Check sheet for the modelled part. Datum: model origin and axes. Units: mm. Round coordinates to 2 decimals unless told otherwise and drop trailing zeros. Write each loop counter-clockwise with the first axis right and the second up, starting at its lowest first coordinate (ties: lowest second). Pieces come first, ordered by that corner, then holes.
Autodesk Inventor part; units mm, degrees
ref_plane "YZ Plane" through (0, 0, 0) normal (1, 0, 0) x (0, 1, 0)
ref_plane "XZ Plane" through (0, 0, 0) normal (0, 1, 0) x (-1, 0, 0)
ref_plane "XY Plane" through (0, 0, 0) normal (0, 0, 1) x (1, 0, 0)
sketch "Sketch1" plane through (0, 0, 0) normal (0, 0, 1) x (1, 0, 0)
  arc A0 (-19.4827, -3.287) -> (-19.05, 0) centre (-31.75, 0) ccw
  line L0 (-19.4827, -3.287) -> (-58.7375, -149.7878)
  line L1 (-65.8876, 46.8376) -> (-65.8876, 21.4376)
  line L2 (-65.8876, 21.4376) -> (-71.4375, 21.4376)
  line L3 (-44.45, 34.1376) -> (-38.6524, 34.1376)
  line L4 (-44.45, 34.1376) -> (0, 34.1376) construction
  line L5 (-37.3992, -46.4536) -> (-31.0492, -46.4536)
  line L6 (-71.4375, 21.4376) -> (-71.4375, 8.7376)
  line L7 (-71.4375, 8.7376) -> (-58.7375, 8.7376)
  line L8 (-58.7375, 8.7376) -> (-52.3875, 8.7376)
  line L9 (-52.3875, 8.7376) -> (-52.3875, -102.3907)
  line L10 (-71.4375, 8.7376) -> (-71.4375, -0.7874)
  line L11 (-71.4375, 8.7376) -> (-61.9125, 8.7376) construction
  line L12 (-71.4375, -0.7874) -> (-58.7375, -0.7874)
  line L13 (-58.7375, -0.7874) -> (-58.7375, -51.5874)
  line L14 (-58.7375, -51.5874) -> (-71.4375, -51.5874)
  line L15 (-71.4375, -0.7874) -> (-65.0875, -0.7874)
  line L16 (-65.0875, -0.7874) -> (-65.0875, -6.731)
  line L17 (-65.0875, -6.731) -> (-71.4375, -6.731)
  line L18 (-71.4375, 21.4376) -> (-71.4375, -0.7874)
  line L19 (-71.4375, -6.731) -> (-71.4375, -51.5874)
  line L20 (-58.7375, -51.5874) -> (-58.7375, -126.0892)
  line L21 (-58.7375, -51.5874) -> (0, -51.5874) construction
  line L22 (-46.0375, -102.3907) -> (-52.3875, -102.3907)
  line L23 (-65.0875, -51.5907) -> (-58.7375, -51.5907)
  line L24 (-58.7375, -149.7878) -> (-61.9125, -161.637)
  line L25 (-58.7375, -149.7878) -> (-34.203, -149.7878) construction
  line L26 (-65.0875, -161.637) -> (-61.9125, -161.637)
  line L27 (-58.7375, -126.0892) -> (-52.3875, -126.0892)
  line L28 (0, 34.1376) -> (0, 0)
  line L29 (-65.0875, -100.6892) -> (-65.0875, -161.637)
  line L30 (-58.7375, -51.5907) -> (-61.9125, -51.5907)
  line L31 (-65.0875, -100.6892) -> (-58.7375, -100.6892)
  line L32 (-65.8876, 46.8376) -> (-18.3062, 46.8376) construction
  line L33 (-65.8876, 46.8376) -> (-14.7047, 46.8376) construction
  line L34 (-65.8876, 46.8376) -> (-33.5957, 31.7796)
  line L35 (-65.8876, 46.8376) -> (-30.2574, 46.8376) construction
  arc A1 (-19.05, 0) -> (-33.5957, 31.7796) centre (-61.0391, 0) ccw
  line L36 (-44.45, 34.1376) -> (-44.45, -46.4536)
  line L37 (-44.45, 34.1376) -> (36.1412, 34.1376) construction
  line L38 (-44.45, -46.4536) -> (-37.3992, -46.4536)
  dimension "d56" = 19.05
  dimension "d57" = 25.4
  dimension "d58" = 5.5499
  dimension "d59" = 65.8876
  dimension "d60" = 12.7
  dimension "d61" = 12.7
  dimension "d62" = 44.45
  dimension "d63" = 6.35
  dimension "d64" = 105
  dimension "d65" = 12.7
  dimension "d66" = 12.7
  dimension "d67" = 6.35
  dimension "d68" = 9.525
  dimension "d69" = 50.8
  dimension "d70" = 12.7
  dimension "d71" = 6.35
  dimension "d72" = 5.9436
  dimension "d73" = 6.35
  dimension "d74" = 50.8
  dimension "d75" = 6.35
  dimension "d76" = 105
  dimension "d77" = 3.175
  dimension "d78" = 6.35
  dimension "d79" = 60.9478
  dimension "d80" = 3.175
  dimension "d81" = 6.35
  dimension "d82" = 25.4
  dimension "d83" = 25
  dimension "d84" = 41.9891
  dimension "d85" = 32.2919
  dimension "d86" = 90
  dimension "d87" = 80.5912
revolve "Revolution1" add sketch "Sketch1" angle 360 about axis through (0, 34.1376, 0) along (0, -1, 0) contours L0 L5 L38 L36 L3 L34 A1 A0
properties part number "Graphite" material "GFRC"
1. Sectioned sample at D-D, the plane y = 20. Enter the section's corners in (x, z), plus the area to 3 significant figures.
2. Sectioned sample at B-B, the plane x = 0. Enter the section's corners in (y, z), plus the area to 3 significant figures.
3. Sectioned sample at C-C, the plane y = -7. Enter the section's corners in (x, z).
4. Release check for a two-part mould opening along Z. For faces 1 (the conical face through (5.2, -20.4, 23.5)), 2 (the cylindrical face through (-42.397, -6.722, -13.352)), 3 (the flat face through (30, -46.454, 9)) record: released by +Z, released by -Z, zero draft, split by the parting line, or undercut.
5. Go/stop test with flat-tipped pins: pin 1 (4 mm diameter, centred on y = -10, z = -15, fed in from -X); pin 2 (1 mm diameter, centred on x = 28.5, y = -36, fed in from -Z); pin 3 (4 mm diameter, centred on x = -21.5, y = -13, fed in from -Z); pin 4 (1.5 mm diameter, centred on x = -35, z = 15, fed in from +Y). Record where each tip stops, or that it passes through.
6. Sectioned sample at A-A, the plane z = 0. Enter the section's corners in (x, y), plus the area to 3 significant figures.
7. Scan lines: line 1 along Z through (x, y) = (-3.5, 1.5); line 2 along Z through (x, y) = (-5.5, -9); line 3 along X through (y, z) = (-23, 11). Record each from-to range of solid material in increasing order.
Computed values:
1. outline: circle Ø88.9 at (0, 0); hole circle Ø48.24 at (0, 0)
1. area: 4,380 mm2
2. outline: (-46.45, -44.45) - (34.14, -44.45) - (34.14, -38.65) - (31.78, -33.6) arc R41.99 ccw to (0, -19.05) arc R12.7 ccw to (-3.29, -19.48) - (-46.45, -31.05) - close; (-46.45, 31.05) - (-3.29, 19.48) arc R12.7 ccw to (0, 19.05) arc R41.99 ccw to (31.78, 33.6) - (34.14, 38.65) - (34.14, 44.45) - (-46.45, 44.45) - close
2. area: 3,190 mm2
3. outline: circle Ø88.9 at (0, 0); hole circle Ø40.96 at (0, 0)
4. face 1: undercut
4. face 2: split by the parting line
4. face 3: zero draft
5. pin 1: stops at x = -42.51
5. pin 2: stops at z = -34.52
5. pin 3: stops at z = -39.94
5. pin 4: stops at y = 34.14
6. outline: (-44.45, -46.45) - (-31.05, -46.45) - (-19.48, -3.29) arc R12.7 ccw to (-19.05, 0) arc R41.99 ccw to (-33.6, 31.78) - (-38.65, 34.14) - (-44.45, 34.14) - close; (19.05, 0) arc R12.7 ccw to (19.48, -3.29) - (31.05, -46.45) - (44.45, -46.45) - (44.45, 34.14) - (38.65, 34.14) - (33.6, 31.78) arc R41.99 ccw to start
6. area: 3,190 mm2
7. line 1: z = -44.31 to -18.75, 18.75 to 44.31
7. line 2: z = -44.11 to -20.28, 20.28 to 44.11
7. line 3: x = -43.07 to -22.19, 22.19 to 43.07
